Input: part model. Units: mm. Frame: model coordinates. A direction names the side the tool comes from. Round coordinates to 2 decimals unless told otherwise and drop trailing zeros. Answer as CSV lines item,"result". Start each with the question number.
```python
from build123d import *

# Parameters (mm, degrees)
F0_W     = 370
F0_H     = 20
F1_DEPTH = 10
F3_DEPTH = 370.001


with BuildPart() as f1:
    # F0 (on Top) → F1 (new body, symmetric)
    with BuildSketch(Plane.XY):
        Rectangle(F0_W, F0_H)
    extrude(amount=F1_DEPTH, both=True)

    # F2 (on face) → F3 (cut, through all)
    with BuildSketch(Plane.YZ.offset(185)):
        Polygon((-8.5, 3), (-10, 4.5), (-10, -4.5), (-8.5, -3), (-8.5, -7.5), (-4.5, -3.5), (-4.5, 0), (-4.5, 3.5), (-8.5, 7.5), align=None)
        Polygon((-3, -8.5), (-4.5, -10), (4.5, -10), (3, -8.5), (7.5, -8.5), (3.5, -4.5), (0, -4.5), (-3.5, -4.5), (-7.5, -8.5), align=None)
        Polygon((10, -4.5), (10, 4.5), (8.5, 3), (8.5, 7.5), (4.5, 3.5), (4.5, 0), (4.5, -3.5), (8.5, -7.5), (8.5, -3), align=None)
        Polygon((4.5, 10), (-4.5, 10), (-3, 8.5), (-7.5, 8.5), (-3.5, 4.5), (0, 4.5), (3.5, 4.5), (7.5, 8.5), (3, 8.5), align=None)
    extrude(amount=-F3_DEPTH, mode=Mode.SUBTRACT)


solid = f1.part
```
Item 1: Pin query (flat end, axial travel): pin 1 Ø5.5 at (x, y) = (-61, -1.5) entering from +Z; pin 2 Ø3.5 at (x, z) = (47.5, 0.5) entering from +Y; pin 3 Ø1.5 at (y, z) = (-4, 6) entering from -X; pin 4 Ø2 at (x, y) = (86, 0.5) entering from -Z. Return the tip coordinate at first contact, or that it passes through.
Item 2: Draft query along Z for faces 3 (the face through (-185, 0, 0)), 4 (the face through (3, 4.5, 0)). Return one class per face: +Z half, -Z half, draft (parallel to the pull), parting line (faces both ways), or undercut.
Item 3: Line query: line 1 (Z direction, x = -137.5, y = 5.25); line 2 (Y direction, x = -21, z = 6); line 3 (Z direction, x = 128, y = -7). Output: solid intervals per line, ascending. Write a range as [from, to].
Item 4: Access query for faces 1 (the face through (185, 0, 0)), 2 (the face through (3, 0, -4.5)). Directions: +Z, -Z, +X, -X, +Y, -Y. A direction counts if a zero-diameter tool reaches every point of the face in a straight line with its end or side. Return the directions, or none.
Results list:
1,pin 1,"z = 9.75"
1,pin 2,"y = 4.5"
1,pin 3,"x = -185"
1,pin 4,"z = -4.5"
2,face 3,"draft"
2,face 4,"undercut"
3,line 1,"[-10, -8.5], [-6.25, -4.25], [4.25, 6.25], [8.5, 10]"
3,line 2,"[-10, -8.5], [-7, -5], [5, 7], [8.5, 10]"
3,line 3,"[-10, -8.5], [-8, -6], [6, 8], [8.5, 10]"
4,face 1,"+Z, -Z, +X, +Y, -Y"
4,face 2,"+X, -X"
